```python
from build123d import *

# Parameters (mm, degrees)
F0_W        = 40.6
F0_H        = 25
F1_DEPTH    = 2
F2_DEPTH    = 30
F3_DEPTH    = 4
F4_DEPTH    = 30
F0_W_2      = 10
F5_DEPTH    = 4
F6_T1_DEPTH = 202.1185772835


# Not quite as in the source:
# - a fillet or chamfer that OpenCascade refuses, or shapes differently, is made with other operations: its cross-section is extruded or revolved along the edge and cut away or added


with BuildPart() as f1:
    # F0 (on Top) → F1 (new body)
    with BuildSketch(Plane.XY):
        with Locations((24.0341860496, -16.1564178318)):
            Rectangle(F0_W, F0_H)
    extrude(amount=F1_DEPTH)

    # F0 (on Top) → F2 (join)
    with BuildSketch(Plane.XY):
        Polygon((44.3341860496, -1.6564178318), (44.3341860496, -3.6564178318), (44.3341860496, -28.6564178318), (44.3341860496, -30.6564178318), (46.3341860496, -30.6564178318), (46.3341860496, -1.6564178318), align=None)
    extrude(amount=F2_DEPTH)

    # F0 (on Top) → F3 (join)
    with BuildSketch(Plane.XY):
        Polygon((44.3341860496, -28.6564178318), (3.7341860496, -28.6564178318), (-6.2658139504, -28.6564178318), (-6.2658139504, -30.6564178318), (44.3341860496, -30.6564178318), align=None)
    extrude(amount=F3_DEPTH)

    # F0 (on Top) → F4 (join)
    with BuildSketch(Plane.XY):
        Polygon((-6.2658139504, -3.6564178318), (3.7341860496, -3.6564178318), (44.3341860496, -3.6564178318), (44.3341860496, -1.6564178318), (-6.2658139504, -1.6564178318), align=None)
    extrude(amount=F4_DEPTH)

    # F0 (on Top) → F5 (join)
    with BuildSketch(Plane.XY):
        with Locations((-1.2658139504, -16.1564178318)):
            Rectangle(F0_W_2, F0_H)
    extrude(amount=F5_DEPTH)

    # F6: fillet of radius 41.6982966493 on 1 edges, made by hand

    # F6_s2 → F6_t1 (cut)
    with BuildSketch(Plane.XZ.offset(-98.40287081)):
        with BuildLine():
            ThreePointArc((-6.2658139504, 0), (8.7484143116, 21.6674566572), (33.7579015062, 30))
            Line((33.7579015062, 30), (-6.2658139504, 30))
            Line((-6.2658139504, 30), (-6.2658139504, 0))
        make_face()
    extrude(amount=F6_T1_DEPTH, mode=Mode.SUBTRACT)


solid = f1.part
```
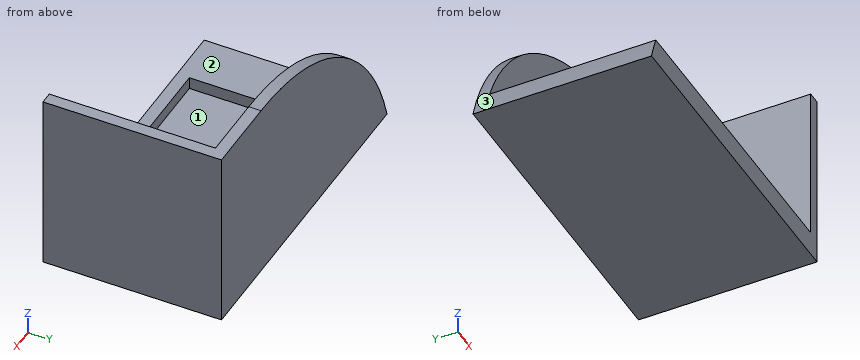
The listing builds one solid part. Answer for the finished solid, in the listing's coordinates (mm). Face numbers are marked on the shaded views. Give positions to 0.01 mm unless a question says otherwise; leave off trailing zeros. Loops run counter-clockwise (first coordinate to the right, second up) from the corner with the lowest first, then second, coordinate; pieces in that order, holes last. Notation, with made-up numbers: M 67,58.5 L 100,58.5 A5 ccw 100,65.5 Z; hole C -38,-35.5 d8. An arc over 180 degrees is marked long. One line per item, written item: value.
1. Each of these flat-tipped pins is pushed along its axis until it touches: P1, Ø5, axis at x = 36, y = -12.5, coming from the +Z side; P2, Ø5, axis at x = 20, z = 22, coming from the -Y side; P3, Ø2, axis at y = -16.5, z = 11.5, coming from the -X side. Where does it stop, or does it pass through?
Found:
P1: z = 2
P2: y = -3.66
P3: x = 44.33
2. For a pull along X with two mould halves and no side action, classify the marked faces 1, 2 and 3 as pulls with the +X half, pulls with the -X half, needs draft (parallel to the pull), parting line crosses it, or undercut.
Found:
face 1: undercut
face 2: needs draft
face 3: pulls with the -X half
3. Find the intervals of material crossed by probe 1 along X at (y, z) = (-20, 23); probe 2 along Z at (x, y) = (11, -29); probe 3 along Y at (x, z) = (29, 11.5), in increasing order.
Found:
probe 1: 44.33 to 46.33
probe 2: 0 to 4
probe 3: -3.66 to -1.66
4. Section D-D on z = 20 is taken. Determine the outline of the cut face in (x, y), plus the area to 3 significant figures.
Found:
outline: M 6.67,-3.66 L 44.33,-3.66 L 44.33,-30.66 L 46.33,-30.66 L 46.33,-1.66 L 6.67,-1.66 Z
area: 133 mm^2
5. Section B-B on x = 8.5 is taken. Determine the outline of the cut face in (y, z).
Found:
outline: M -30.66,0 L -1.66,0 L -1.66,21.48 L -3.66,21.48 L -3.66,2 L -28.66,2 L -28.66,4 L -30.66,4 Z
6. Section C-C on z = 3 is taken. Determine the outline of the cut face in (x, y), plus the area to 3 significant figures.
Found:
outline: M -5.26,-30.66 L 46.33,-30.66 L 46.33,-1.66 L -5.26,-1.66 Z; hole M 3.73,-28.66 L 44.33,-28.66 L 44.33,-3.66 L 3.73,-3.66 Z
area: 481 mm^2
7. Section A-A on y = -21.75 is taken. Determine the outline of the cut face in (x, z), plus the area to 3 significant figures.
Found:
outline: M -6.27,0 L 46.33,0 L 46.33,30 L 44.33,30 L 44.33,2 L 3.73,2 L 3.73,4 L -4.87,4 A41.7 ccw Z
area: 179 mm^2
